Build history of the part. All positions in model axes, mm. Round coordinates to 2 decimals unless told otherwise and drop trailing zeros. Write each loop counter-clockwise with the first axis right and the second up, starting at its lowest first coordinate (ties: lowest second). Pieces come first, ordered by that corner, then holes. Notation, with made-up numbers: (-22, 9.5) - (32, 9.5) arc R8 ccw to (32, 13.5) - close; hole circle Ø4 at (-5, -30.5). An arc over 180 degrees is marked (long way). Answer as a JSON object with one key per item and string values. Group by question number.
Item 1: Flat gauge pin, fed straight in: pin 1 (1.8 mm diameter, centred on x = -25, y = -0.75, fed in from +Z). Where does the tip first touch, or does it go through?
Item 2: Slice it at D-D, the plane y = -4.5. List the corners of the cut face in (x, z), then the cut area to 3 significant figures.
Item 3: Slice it at C-C, the plane z = 0.8. List the corners of the cut face in (x, y), then the cut area to 3 significant figures.
Item 4: Slice it at A-A, the plane x = -25. List the corners of the cut face in (y, z).
Item 5: Probe line 1 (Y direction, x = 25, z = 2.15); line 2 (X direction, y = -1.25, z = 1.4); line 3 (X direction, y = -2, z = 1.75). List the from-to ranges inside material, lowest first. Write a range as from..to.
Item 6: Slice it at B-B, the plane y = -0.75. List the corners of the cut face in (x, z), then the cut area to 3 significant figures.
from build123d import *

# Parameters (mm, degrees)
SKETCH1_R           = 1.5
BOSS_EXTRUDE1_DEPTH = 3


with BuildPart() as part:
    # Sketch1 → Boss-Extrude1 (new body)
    with BuildSketch(Plane.XY):
        with BuildLine():
            Line((-31, 2.5), (31, 2.5))
            Line((31, 2.5), (31, -2.5))
            ThreePointArc((31, -2.5), (30.121320344, -4.621320344), (28, -5.5))
            Line((28, -5.5), (-28, -5.5))
            ThreePointArc((-28, -5.5), (-30.121320344, -4.621320344), (-31, -2.5))
            Line((-31, -2.5), (-31, 2.5))
        make_face()
        with Locations((-25, -0.75)):
            Circle(SKETCH1_R, mode=Mode.SUBTRACT)
        with Locations((25, -0.75)):
            Circle(SKETCH1_R, mode=Mode.SUBTRACT)
    extrude(amount=BOSS_EXTRUDE1_DEPTH)


solid = part.part
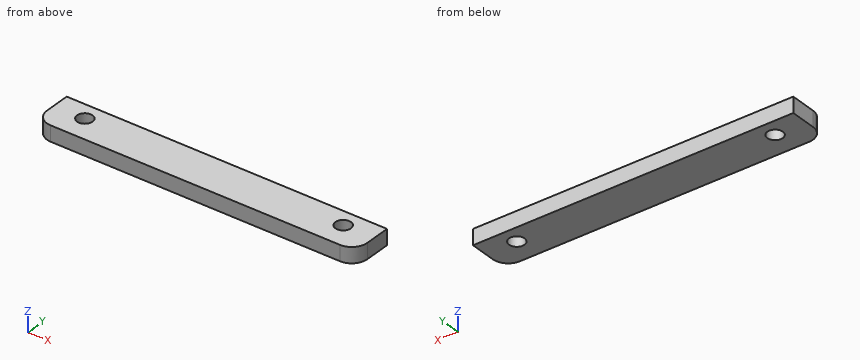
Geometry says:
{
 "1": {"pin 1": "passes through"},
 "2": {"outline": "(-30.24, 0) - (30.24, 0) - (30.24, 3) - (-30.24, 3) - close", "area": "181 mm^2"},
 "3": {"outline": "(-31, -2.5) arc R3 ccw to (-28, -5.5) - (28, -5.5) arc R3 ccw to (31, -2.5) - (31, 2.5) - (-31, 2.5) - close; hole circle Ø3 at (-25, -0.75); hole circle Ø3 at (25, -0.75)", "area": "478 mm^2"},
 "4": {"outline": "(-5.5, 0) - (-2.25, 0) - (-2.25, 3) - (-5.5, 3) - close; (0.75, 0) - (2.5, 0) - (2.5, 3) - (0.75, 3) - close"},
 "5": {"line 1": "y = -5.5..-2.25, 0.75..2.5", "line 2": "x = -31..-26.41, -23.59..23.59, 26.41..31", "line 3": "x = -31..-25.83, -24.17..24.17, 25.83..31"},
 "6": {"outline": "(-31, 0) - (-26.5, 0) - (-26.5, 3) - (-31, 3) - close; (-23.5, 0) - (23.5, 0) - (23.5, 3) - (-23.5, 3) - close; (26.5, 0) - (31, 0) - (31, 3) - (26.5, 3) - close", "area": "168 mm^2"}
}
